Autodesk Inventor part; units mm, degrees
ref_plane "YZ Plane" through (0, 0, 0) normal (1, 0, 0) x (0, 1, 0)
ref_plane "XZ Plane" through (0, 0, 0) normal (0, 1, 0) x (-1, 0, 0)
ref_plane "XY Plane" through (0, 0, 0) normal (0, 0, 1) x (1, 0, 0)
sketch "Sketch1" plane through (0, 0, 0) normal (0, 1, 0) x (-1, 0, 0)
  line L0 (45, 47.5) -> (-45, 47.5)
  line L1 (-45, 47.5) -> (-45, -47.5)
  line L2 (-45, -47.5) -> (45, -47.5)
  line L3 (45, -47.5) -> (45, 47.5)
  line L4 (45, 47.5) -> (-45, -47.5) construction
  line L5 (-45, 47.5) -> (45, -47.5) construction
  point P0 (0, 0)
  dimension "d0" = 95
  dimension "d1" = 90
extrude "Extrusion1" add sketch "Sketch1" along normal blind 1.45
sketch "Sketch2" plane through (0, 1.45, 0) normal (0, 1, 0) x (1, 0, 0)
  circle A0 centre (37.38, 42.42) radius 1.75
  circle A1 centre (-40.09, -43.305) radius 1.75
  circle A2 centre (39.92, -43.305) radius 1.75
  circle A3 centre (-36.28, 42.42) radius 1.75
  line L0 (-45, 47.5) -> (-45, -47.5)
  line L1 (45, 47.5) -> (-45, 47.5)
  line L2 (45, -47.5) -> (45, 47.5)
  point P0 (0, 0)
  dimension "d4" = 3.5
  dimension "d5" = 3.5
  dimension "d6" = 3.5
  dimension "d7" = 3.5
  dimension "d46" = 73.66
  dimension "d47" = 7.62
  dimension "d48" = 5.08
  dimension "d49" = 85.725
  dimension "d50" = 80.01
  dimension "d51" = 2.54
extrude "Extrusion2" cut sketch "Sketch2" against normal through all
sketch "Sketch3" plane through (0, 1.45, 0) normal (0, 1, 0) x (1, 0, 0)
  circle A0 centre (-36.28, 42.42) radius 1.75
  circle A1 centre (11.98, 41.15) radius 1.75
  line L0 (45, 47.5) -> (-45, 47.5)
  circle A2 centre (-31.2, -9.65) radius 1.75
  circle A3 centre (-36.28, 42.42) radius 1.75
  point P0 (0, 0)
  dimension "d18" = 3.5
  dimension "d19" = 3.5
  dimension "d22" = 48.26
  dimension "d23" = 1.27
  dimension "d24" = 3.5
  dimension "d25" = 5.08
  dimension "d26" = 52.07
  dimension "d44" = 0
  dimension "d45" = 0
extrude "Extrusion3" cut sketch "Sketch3" against normal blind 10
sketch "Sketch4" plane through (0, 1.45, 0) normal (0, 1, 0) x (1, 0, 0)
  line L0 (-36.28, 27.42) -> (-36.28, -7.58) construction
  line L1 (-38.03, 27.42) -> (-38.03, -7.58)
  line L2 (-34.53, -7.58) -> (-34.53, 27.42)
  arc A0 (-34.53, 27.42) -> (-38.03, 27.42) centre (-36.28, 27.42) ccw
  arc A1 (-38.03, -7.58) -> (-34.53, -7.58) centre (-36.28, -7.58) ccw
  line L3 (11.98, 36.65) -> (11.98, -8.35) construction
  line L4 (10.23, 36.65) -> (10.23, -8.35)
  line L5 (13.73, -8.35) -> (13.73, 36.65)
  arc A2 (13.73, 36.65) -> (10.23, 36.65) centre (11.98, 36.65) ccw
  arc A3 (10.23, -8.35) -> (13.73, -8.35) centre (11.98, -8.35) ccw
  circle A4 centre (-36.28, 42.42) radius 1.75
  circle A5 centre (11.98, 41.15) radius 1.75
  line L6 (-23.58, 36.67) -> (-23.58, 14.67) construction
  line L7 (-25.33, 36.67) -> (-25.33, 14.67)
  line L8 (-21.83, 14.67) -> (-21.83, 36.67)
  arc A6 (-21.83, 36.67) -> (-25.33, 36.67) centre (-23.58, 36.67) ccw
  arc A7 (-25.33, 14.67) -> (-21.83, 14.67) centre (-23.58, 14.67) ccw
  line L9 (-0.72, 36.67) -> (-0.72, 14.67) construction
  line L10 (-2.47, 36.67) -> (-2.47, 14.67)
  line L11 (1.03, 14.67) -> (1.03, 36.67)
  arc A8 (1.03, 36.67) -> (-2.47, 36.67) centre (-0.72, 36.67) ccw
  arc A9 (-2.47, 14.67) -> (1.03, 14.67) centre (-0.72, 14.67) ccw
  line L12 (-31.2, 42.5) -> (-31.2, 29.8) construction
  line L13 (-32.7, 42.5) -> (-32.7, 29.8)
  line L14 (-29.7, 29.8) -> (-29.7, 42.5)
  arc A10 (-29.7, 42.5) -> (-32.7, 42.5) centre (-31.2, 42.5) ccw
  arc A11 (-32.7, 29.8) -> (-29.7, 29.8) centre (-31.2, 29.8) ccw
  line L15 (45, 47.5) -> (-45, 47.5)
  line L16 (-45, 47.5) -> (-45, -47.5)
  point P0 (0, 0)
  point P1 (-36.28, 9.92)
  point P2 (11.98, 14.15)
  point P3 (-23.58, 25.67)
  point P4 (-0.72, 25.67)
  point P5 (-23.58, 38.42)
  point P6 (-31.2, 36.15)
  dimension "d28" = 3.5
  dimension "d29" = 3.5
  dimension "d30" = 15
  dimension "d31" = 35
  dimension "d32" = 4.5
  dimension "d33" = 45
  dimension "d34" = 12.7
  dimension "d35" = 35.56
  dimension "d36" = 3.5
  dimension "d37" = 3.5
  dimension "d38" = 22
  dimension "d41" = 4
  dimension "d52" = 3
  dimension "d53" = 5
  dimension "d54" = 12.7
  dimension "d56" = 5.08
extrude "Extrusion4" cut sketch "Sketch4" against normal blind 10 contours A0 L2 A1 L1 | A2 L5 A3 L4 | A6 L8 A7 L7 | A8 L11 A9 L10 | A10 L14 A11 L13
properties part number "empty_board" material "ABS Plastic"
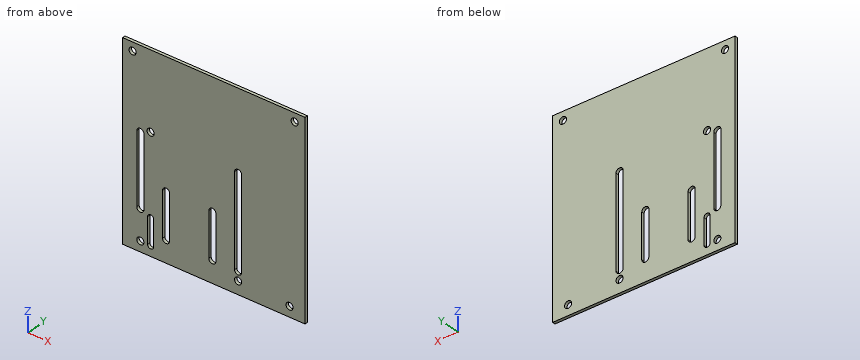
Geometry: final body of the model. Coordinates: model frame, mm. Coordinates: 2 decimals unless noted, no trailing zeros. Order: outer loops, then holes, each group sorted by start corner. A loop starts at its lowest first (then second) coordinate and runs counter-clockwise, first axis right, second up. Notation, with made-up numbers: (62, 32) -> (70, 32) arc R16 cw to (70, 54) -> close; hole circle Ø7 at (7.5, -26.5). An arc over 180 degrees is marked (long way). Use CSV: the item, a comma, the result in double quotes.
1) Line query: line 1 (X direction, y = 0.85, z = -30); line 2 (X direction, y = 0.3, z = -16); line 3 (X direction, y = 0.75, z = 43). Output: solid intervals per line, ascending.
Findings:
line 1,"x = -45 to -32.7, -29.7 to -25.33, -21.83 to -2.47, 1.03 to 10.23, 13.73 to 45"
line 2,"x = -45 to -38.03, -34.53 to -25.33, -21.83 to -2.47, 1.03 to 10.23, 13.73 to 45"
line 3,"x = -45 to -41.81, -38.37 to 38.2, 41.64 to 45"
2) Pin query (flat end, axial travel): pin 1 Ø3 at (x, z) = (11.98, -41.15) entering from -Y; pin 2 Ø5.5 at (x, z) = (39.92, 43.305) entering from +Y. Return the tip coordinate at first contact, or that it passes through.
Findings:
pin 1,"passes through"
pin 2,"stops at y = 1.45"
3) Section B-B on x = -36.28. Output: boundary loops of the cut face in (y, z).
Findings:
outline,"(0, -47.5) -> (1.45, -47.5) -> (1.45, -44.17) -> (0, -44.17) -> close; (0, -40.67) -> (1.45, -40.67) -> (1.45, -29.17) -> (0, -29.17) -> close; (0, 9.33) -> (1.45, 9.33) -> (1.45, 47.5) -> (0, 47.5) -> close"
4) Section D-D on x = -0.72. Output: boundary loops of the cut face in (y, z), then the cut area to 3 significant figures.
Findings:
outline,"(0, -47.5) -> (1.45, -47.5) -> (1.45, -38.42) -> (0, -38.42) -> close; (0, -12.92) -> (1.45, -12.92) -> (1.45, 47.5) -> (0, 47.5) -> close"
area,"101 mm^2"
5) Section A-A on z = -21.5. Output: boundary loops of the cut face in (x, y), then the cut area to 3 significant figures.
Findings:
outline,"(-45, 0) -> (-38.03, 0) -> (-38.03, 1.45) -> (-45, 1.45) -> close; (-34.53, 0) -> (-25.33, 0) -> (-25.33, 1.45) -> (-34.53, 1.45) -> close; (-21.83, 0) -> (-2.47, 0) -> (-2.47, 1.45) -> (-21.83, 1.45) -> close; (1.03, 0) -> (10.23, 0) -> (10.23, 1.45) -> (1.03, 1.45) -> close; (13.73, 0) -> (45, 0) -> (45, 1.45) -> (13.73, 1.45) -> close"
area,"110 mm^2"
6) Section C-C on z = -9. Output: boundary loops of the cut face in (x, y).
Findings:
outline,"(-45, 0) -> (-38.03, 0) -> (-38.03, 1.45) -> (-45, 1.45) -> close; (-34.53, 0) -> (10.23, 0) -> (10.23, 1.45) -> (-34.53, 1.45) -> close; (13.73, 0) -> (45, 0) -> (45, 1.45) -> (13.73, 1.45) -> close"
